from build123d import *

# Parameters (mm, degrees)
F0_R      = 1.625
F0_R_2    = 5.1
F1_DEPTH  = 65
F2_W      = 20.1791324483
F2_H      = 55
F3_DEPTH  = 19.001
F4_R      = 15.5
F4_R_2    = 1.5
F5_DEPTH  = 18.001
F6_R      = 4
F7_DEPTH  = 40
F13_DEPTH = 4
F14_W     = 20
F14_H     = 27.55
F15_DEPTH = 10
F16_DEPTH = 2.5
F17_R     = 1.6
F18_DEPTH = 62.501


with BuildPart() as f1:
    # F0 (on Top) → F1 (new body)
    with BuildSketch(Plane.XY):
        with BuildLine():
            Line((0, 0), (0, 18))
            Line((0, 18), (-90, 18))
            Line((-90, 18), (-90, 0))
            Line((-90, 0), (-41.5, 0))
            Line((-41.5, 0), (-41.5, -7.5))
            Line((-41.5, -7.5), (-37.5, -7.5))
            ThreePointArc((-37.5, -7.5), (-22.5167601334, -6.9988801553), (-37.4330343737, -8.5))
            Line((-37.4330343737, -8.5), (-41.4564392374, -8.5))
            ThreePointArc((-41.4564392374, -8.5), (-34.6794450635, -18.0048938071), (-23.0807416268, -16.6855246755))
            ThreePointArc((-23.0807416268, -16.6855246755), (-20.1791324483, -15.6803710419), (-17.2372532895, -16.5607213511))
            ThreePointArc((-17.2372532895, -16.5607213511), (-5.8818844378, -17.2367804274), (0, -7.5))
            Line((0, -7.5), (0, 0))
        make_face()
        with Locations((-11, -15.5)):
            Circle(F0_R, mode=Mode.SUBTRACT)
        with Locations((-19, -7.5)):
            Circle(F0_R, mode=Mode.SUBTRACT)
        with Locations((-11, -7.5)):
            Circle(F0_R_2, mode=Mode.SUBTRACT)
        with Locations((-3, -7.5)):
            Circle(F0_R, mode=Mode.SUBTRACT)
    extrude(amount=F1_DEPTH)

    # F2 (on face) → F3 (cut, through all)
    with BuildSketch(Plane.XZ):
        with Locations((-10.0895662241, 27.5)):
            Rectangle(F2_W, F2_H)
    extrude(amount=F3_DEPTH, mode=Mode.SUBTRACT)

    # F4 (on face) → F5 (cut, through all)
    with BuildSketch(Plane.XZ):
        with Locations((-67, 32.5)):
            Circle(F4_R)
        with Locations((-82.5, 17)):
            Circle(F4_R_2)
        with Locations((-51.5, 17)):
            Circle(F4_R_2)
        with Locations((-51.5, 48)):
            Circle(F4_R_2)
        with Locations((-82.5, 48)):
            Circle(F4_R_2)
    extrude(amount=-F5_DEPTH, mode=Mode.SUBTRACT)

    # F6 (on face) → F7 (cut)
    with BuildSketch(Plane.YZ):
        with Locations((9, 58)):
            Circle(F6_R)
        with Locations((9, 7)):
            Circle(F6_R)
    extrude(amount=-F7_DEPTH, mode=Mode.SUBTRACT)

    # F12 (on 3pt) → F13 (cut, symmetric)
    with BuildSketch(Plane.XZ.offset(-9)):
        with BuildLine():
            Line((-67, 32.5), (0, 32.5))
            Line((0, 32.5), (0, 47.5))
            Line((0, 47.5), (-41.4564392374, 47.5))
            ThreePointArc((-41.4564392374, 47.5), (-44.6149693804, 46.7572666031), (-47.1114866019, 44.6847398058))
            ThreePointArc((-47.1114866019, 44.6847398058), (-49.0488707774, 43.0763869431), (-51.5, 42.5))
            Line((-51.5, 42.5), (-67, 42.5))
            Line((-67, 42.5), (-67, 32.5))
        make_face()
        with BuildLine():
            Line((0, 17.5), (0, 32.5))
            Line((0, 32.5), (-67, 32.5))
            Line((-67, 32.5), (-67, 22.5))
            Line((-67, 22.5), (-51.5, 22.5))
            ThreePointArc((-51.5, 22.5), (-49.0488707774, 21.9236130569), (-47.1114866019, 20.3152601942))
            ThreePointArc((-47.1114866019, 20.3152601942), (-44.6149693804, 18.2427333969), (-41.4564392374, 17.5))
            Line((-41.4564392374, 17.5), (0, 17.5))
        make_face()
    extrude(amount=F13_DEPTH, both=True, mode=Mode.SUBTRACT)

    # F14 (on face) → F15 (join)
    with BuildSketch(Plane(origin=(0, 0, 0), x_dir=(1, 0, 0), z_dir=(0, 0, -1))):
        with Locations((-56.5, 13.775)):
            Rectangle(F14_W, F14_H)
        Polygon((-52.95, 19), (-54.725, 15.9256098166), (-58.275, 15.9256098166), (-60.05, 19), (-58.275, 22.0743901834), (-54.725, 22.0743901834), align=None, mode=Mode.SUBTRACT)
        Polygon((-71.5, 0), (-66.5, 0), (-66.5, 27.55), align=None)
        Polygon((-46.5, 27.55), (-46.5, 0), (-41.5, 0), align=None)
        Polygon((-58.275, 15.9256098166), (-54.725, 15.9256098166), (-52.95, 19), (-54.725, 22.0743901834), (-58.275, 22.0743901834), (-60.05, 19), align=None)
    extrude(amount=-F15_DEPTH)

    # F14 (on face) → F16 (cut)
    with BuildSketch(Plane(origin=(0, 0, 0), x_dir=(1, 0, 0), z_dir=(0, 0, -1))):
        Polygon((-58.275, 15.9256098166), (-54.725, 15.9256098166), (-52.95, 19), (-54.725, 22.0743901834), (-58.275, 22.0743901834), (-60.05, 19), align=None)
    extrude(amount=-F16_DEPTH, mode=Mode.SUBTRACT)

    # F17 (on face) → F18 (cut, through all)
    with BuildSketch(Plane(origin=(0, 0, 2.5), x_dir=(1, 0, 0), z_dir=(0, 0, -1))):
        with Locations((-56.5, 19)):
            Circle(F17_R)
    extrude(amount=-F18_DEPTH, mode=Mode.SUBTRACT)


solid = f1.part
Source: CAD feature listing. Evaluate the final solid. Frame: model axes, mm. A direction names the side the tool comes from. Coordinates: 2 decimals unless noted, no trailing zeros. Order: outer loops, then holes, each group sorted by start corner. A loop starts at its lowest first (then second) coordinate and runs counter-clockwise, first axis right, second up. Notation, with made-up numbers: M -13,-12 L 9,-12 A38 ccw 9,27 Z; hole C -12.5,38 d10. An arc over 180 degrees is marked long. Write each question's results on one line, items separated by ' | '. Start each with the question number.
1. Draft query along Z for faces 1 (the face through (-59.15, -20.56, 1.23)), 2 (the face through (-52.61, 8.87, 18.01)), 3 (the face through (-5.7, -9.1, 55)). Return one class per face: +Z half, -Z half, draft (parallel to the pull), parting line (faces both ways), or undercut.
2. Material intervals for L1, parallel to Y at x = -30, z = 18; L2, parallel to Y at x = -31, z = 9.5; L3, parallel to Z at x = -51, y = 12, sorted ascending.
3. Section B-B, the plane z = 12. Return the cut outline in (x, y) (3 decimals).
4. Pin query (flat end, axial travel): pin 1 (12 mm diameter, centred on x = -26, z = 47.5, fed in from -Y); pin 2 (1.5 mm diameter, centred on x = -71.5, z = 55, fed in from -Y); pin 3 (3 mm diameter, centred on y = -4.5, z = 33, fed in from +X); pin 4 (1.8 mm diameter, centred on x = -51.5, z = 48, fed in from +Y). Return the tip coordinate at first contact, or that it passes through.
5. Section D-D, the plane x = -68.5. Return the cut outline in (y, z).
6. Section A-A, the plane x = -30. Return the cut outline in (y, z), then the cut area to 3 significant figures.
7. Reachability of faces 4 (the face through (-77, 0, 46)), 5 (the face through (-59.175, -17.484, 1.232)), 6 (the face through (-20.179, -3, 27)) from +Z, -Z, +X, -X, +Y, -Y: full face, straight path, thin tool, end or side. Return the list, or none.
8. Section C-C, the plane y = -3.5. Return the cut outline in (x, z).
Solution:
1) face 1: draft | face 2: undercut | face 3: -Z half
2) L1: -19 to -15, 0 to 5, 13 to 18 | L2: -18.96 to -14.93, -0.07 to 5.88, 12.12 to 18 | L3: 0 to 15.59, 18.41 to 22.48, 42.52 to 46.59, 49.41 to 65
3) outline: M -90,0 L -41.5,0 L -41.5,-7.5 L -37.5,-7.5 A7.5 cw long -37.433,-8.5 L -41.456,-8.5 A11.5 ccw -23.081,-16.686 A5 cw -20.179,-15.68 L -20.179,-8.618 A1.625 cw -20.179,-6.382 L -20.179,0 L 0,0 L 0,18 L -90,18 Z
4) pin 1: y = -19 | pin 2: y = 0 | pin 3: x = -20.18 | pin 4: through
5) outline: M -16.53,0 L 18,0 L 18,17.07 L 0,17.07 L 0,10 L -16.53,10 Z; M 0,47.93 L 18,47.93 L 18,65 L 0,65 Z
6) outline: M -19,0 L -15,0 L -15,65 L -19,65 Z; M 0,0 L 18,0 L 18,65 L 0,65 Z; hole C 9,7 d8; hole M 5,17.5 L 13,17.5 L 13,47.5 L 5,47.5 Z; hole C 9,58 d8 | area: 1,090 mm²
7) face 4: +Z, -X, -Y | face 5: -Z | face 6: -Z, +X, -Y
8) outline: M -70.86,0 L -42.14,0 L -42.14,10 L -70.86,10 Z; M -41.5,0 L -36.34,0 L -36.34,65 L -41.5,65 Z; M -23.66,0 L -20.18,0 L -20.18,55 L -14.16,55 L -14.16,65 L -23.66,65 Z; M -7.84,55 L 0,55 L 0,65 L -7.84,65 Z
